Study the drawing (mm; zero at the part's minimum x, y, z) and answer. A direction names the side the tool comes from. Coordinates: 2 decimals unless noted, no trailing zeros. Order: outer loops, then holes, each group sorted by start corner. A loop starts at its lowest first (then second) coordinate and runs counter-clockwise, first axis right, second up. Notation, with made-up numbers: M -16,59 L 4,59 A19 cw 4,80 Z; hole C 66.25,-18 d10. An arc over 180 degrees is marked long. Put each result on its own line as item: value.
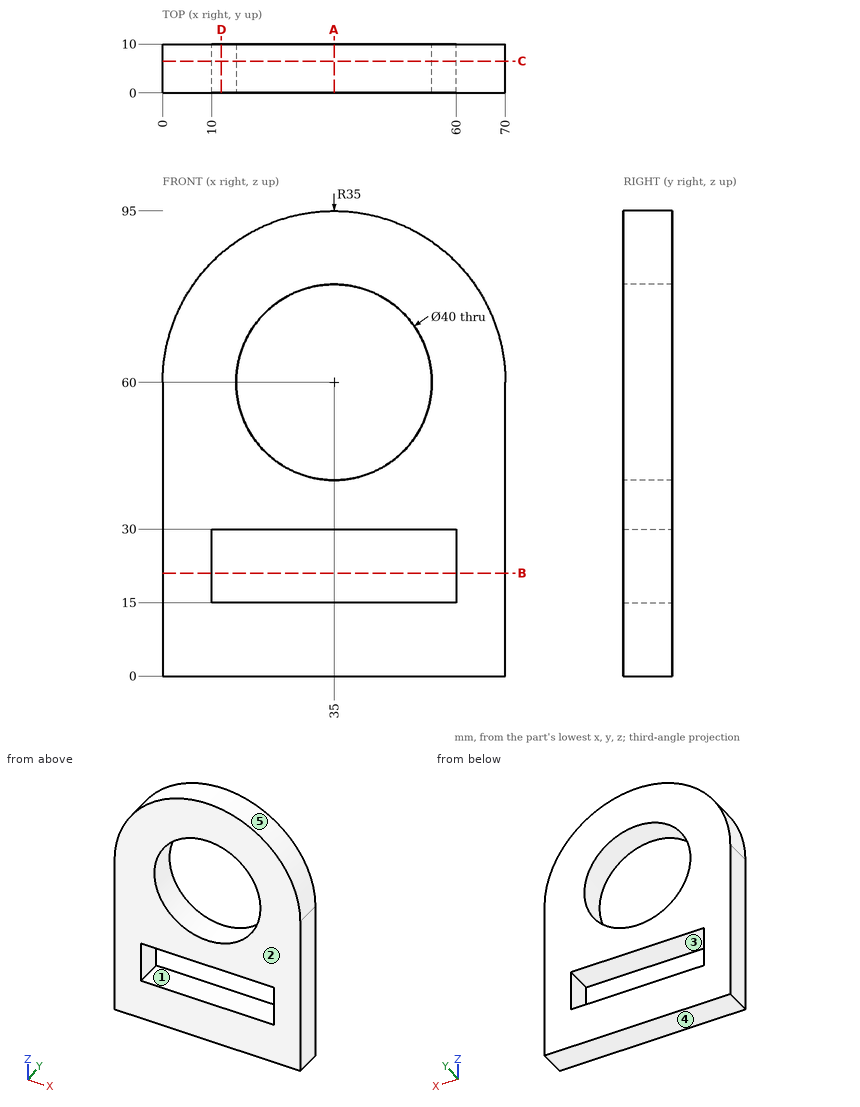
Q1. Find section C-C on y = 6.5. Write down the section's boundary in (x, z), plus the area to 3 significant figures.
Answers below:
outline: M 0,0 L 70,0 L 70,60 A35 ccw 0,60 Z; hole M 10,15 L 60,15 L 60,30 L 10,30 Z; hole C 35,60 d40
area: 4,120 mm^2
Q2. Find section A-A on x = 35. Write down the section's boundary in (y, z), plus the area to 3 significant figures.
Answers below:
outline: M 0,0 L 10,0 L 10,15 L 0,15 Z; M 0,30 L 10,30 L 10,40 L 0,40 Z; M 0,80 L 10,80 L 10,95 L 0,95 Z
area: 400 mm^2
Q3. Given pin 1 (3 mm diameter, centred on x = 50, y = 3.5, fed in from +Z); pin 2 (5 mm diameter, centred on y = 5.5, z = 25, fed in from -X); pin 3 (1 mm diameter, centred on y = 3.5, z = 73.5, fed in from +X); pin 4 (3 mm diameter, centred on x = 20.5, y = 3, fed in from +Z), each flat-ended and moving along its own axis, determine where each tip first touches the part or whether it passes through.
Answers below:
pin 1: stops at z = 92.29
pin 2: stops at x = 0
pin 3: stops at x = 67.5
pin 4: stops at z = 92.5
Q4. Find section B-B on z = 21. Write down the section's boundary in (x, y).
Answers below:
outline: M 0,0 L 10,0 L 10,10 L 0,10 Z; M 60,0 L 70,0 L 70,10 L 60,10 Z
Q5. For a pull along X with two mould halves and no side action, classify the marked faces 3, 4 and 5 as +X half, -X half, draft (parallel to the pull), parting line (faces both ways), or undercut.
Answers below:
face 3: undercut
face 4: draft
face 5: parting line
Q6. Find section D-D on x = 12. Write down the section's boundary in (y, z), plus the area to 3 significant figures.
Answers below:
outline: M 0,0 L 10,0 L 10,15 L 0,15 Z; M 0,30 L 10,30 L 10,86.38 L 0,86.38 Z
area: 714 mm^2
Q7. Consider line 1 along Z through (x, y) = (35, 3.75); line 2 along X through (y, z) = (6.5, 60); line 3 along Z through (x, y) = (36.5, 5.75). Determine where each line is inside the solid, lowest interval first.
Answers below:
line 1: z = 0 to 15, 30 to 40, 80 to 95
line 2: x = 0 to 15, 55 to 70
line 3: z = 0 to 15, 30 to 40.06, 79.94 to 94.97
Q8. A tool of negligible diameter and unlimited length cuts with its end or side. For the marked faces 1 and 2, from which of +Z, -Z, +X, -X, +Y, -Y can it reach the whole face along a straight path? Write none if from no direction.
Answers below:
face 1: +Y, -Y
face 2: +Z, -Z, +X, -X, -Y
